Can you work these out from the model? Positions are in its coordinate system, mm. Face numbers are marked on the shaded views. Give positions to 0.01 mm unless a question says otherwise; leave off trailing zeros. Loops run counter-clockwise (first coordinate to the right, second up) from the corner with the lowest first, then second, coordinate; pieces in that order, holes last. Notation, with made-up numbers: M 59.5,29 L 99.5,29 A27 ccw 99.5,64 Z; hole C 7.25,38.5 d9. An arc over 180 degrees is marked long. Put each result on its own line as item: value. Start each with the question number.
1) Please list where these lines run through material, in increasing order: line 1 along X through (y, z) = (33.5, 2); line 2 along X through (y, z) = (102, 6); line 3 along Y through (x, z) = (59.5, 18.5). Write a range as from..to.
2) For P1, Ø8, axis at y = 116.5, z = 14, coming from the -X side; P2, Ø1, axis at y = 85, z = 14.5, coming from the -X side; P3, Ø12, axis at x = 195.5, z = 8, coming from the +Y side, each with a flat end and sliding along its axis, tell me the tip position at first contact or that it passes through.
3) Imagine slicing it at D-D (y = 90.5). Write out the boundary of the cut face in (x, z).
4) Imagine slicing it at C-C (x = 125). Write out the boundary of the cut face in (y, z), then the cut area to 3 significant figures.
5) If we mould it in two halves opening along X, with no side actions, what happens to the marked faces 1 and 2? For each: +X half, -X half, draft (parallel to the pull), parting line (faces both ways), or undercut.
6) Imagine slicing it at A-A (y = 47.5). Write out the boundary of the cut face in (x, z).
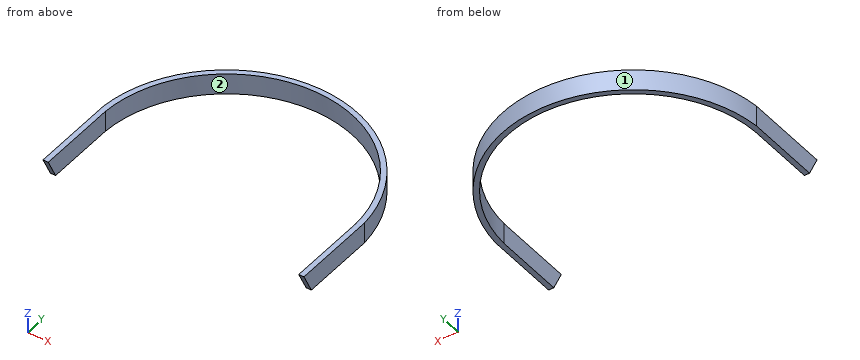
from build123d import *

# Parameters (mm, degrees)
BOSS_EXTRU_1_DEPTH      = 20
ENL_V_MAT_EXTRU_1_DEPTH = 319.918484883


with BuildPart() as part:
    # Esquisse1 → Boss.-Extru.1 (new body)
    with BuildSketch(Plane.XY):
        with BuildLine():
            Line((5, 0), (5, 77))
            ThreePointArc((5, 77), (125, 192), (245, 77))
            Line((245, 77), (245, 0))
            Line((245, 0), (250, 0))
            Line((250, 0), (250, 82))
            ThreePointArc((250, 82), (125, 197), (0, 82))
            Line((0, 82), (0, 0))
            Line((0, 0), (5, 0))
        make_face()
    extrude(amount=BOSS_EXTRU_1_DEPTH)

    # Esquisse2 → Enlèv. mat.-Extru.1 (cut, through all)
    with BuildSketch(Plane(origin=(250, 0, 0), x_dir=(0, 0, -1), z_dir=(1, 0, 0))):
        Polygon((-20, 0), (0, 0), (0, 10), align=None)
    extrude(amount=-ENL_V_MAT_EXTRU_1_DEPTH, mode=Mode.SUBTRACT)


solid = part.part
Recorded:
1. line 1: 0..5, 245..250
1. line 2: 3.31..8.73, 241.27..246.69
1. line 3: 172.57..178.54
2. P1: x = 6.43
2. P2: x = 0.23
2. P3: y = 179.15
3. outline: M 1,0 L 6.34,0 L 6.34,20 L 1,20 Z; M 243.66,0 L 249,0 L 249,20 L 243.66,20 Z
4. outline: M 192,0 L 197,0 L 197,20 L 192,20 Z
4. area: 100 mm²
5. face 1: parting line
5. face 2: undercut
6. outline: M 0,0 L 5,0 L 5,20 L 0,20 Z; M 245,0 L 250,0 L 250,20 L 245,20 Z
